Build history of the part. All positions in model axes, mm. A direction names the side the tool comes from. Coordinates: 2 decimals unless noted, no trailing zeros. Loops run counter-clockwise (first coordinate to the right, second up) from the corner with the lowest first, then second, coordinate; pieces in that order, holes last. Notation, with made-up numbers: M 10,10.5 L 23,10.5 A21 ccw 23,18.5 Z; hole C -27.75,69 d9. An arc over 180 degrees is marked long. Write each question's results on one line, items separated by ' | '. Start each with the question number.
from build123d import *

# Parameters (mm, degrees)
SKETCH1_W           = 120
SKETCH1_H           = 15
BOSS_EXTRUDE1_DEPTH = 5
SKETCH2_W           = 7
SKETCH2_H           = 4
CUT_EXTRUDE1_DEPTH  = 10
CUT_EXTRUDE2_DEPTH  = 7


with BuildPart() as part:
    # Sketch1 → Boss-Extrude1 (new body)
    with BuildSketch(Plane(origin=(0, 0, 0), x_dir=(1, 0, 0), z_dir=(0, 1, 0))):
        with Locations((60, 7.5)):
            Rectangle(SKETCH1_W, SKETCH1_H)
    extrude(amount=BOSS_EXTRUDE1_DEPTH)

    # Sketch2 → Cut-Extrude1 (cut)
    with BuildSketch(Plane(origin=(0, 5, 0), x_dir=(1, 0, 0), z_dir=(0, 1, 0))):
        with Locations((60, 7.5)):
            Rectangle(SKETCH2_W, SKETCH2_H)
    extrude(amount=-CUT_EXTRUDE1_DEPTH, mode=Mode.SUBTRACT)

    # Sketch3 → Cut-Extrude2 (cut)
    with BuildSketch(Plane(origin=(56.5, 0, 0), x_dir=(0, 0, -1), z_dir=(1, 0, 0))):
        Polygon((5.5, 5), (3.997858335, 5), (5.5, 2.5), align=None)
        Polygon((9.5, 5), (11, 5), (9.5, 2.5), align=None)
        Polygon((1.5, 5), (0, 2.5), (0, 5), align=None)
        Polygon((13.5, 5), (15, 2.5), (15, 5), align=None)
    extrude(amount=CUT_EXTRUDE2_DEPTH, mode=Mode.SUBTRACT)


solid = part.part
1. Band-saw the part on B-B, the plane y = 1.2. List the corners of the cut face in (x, z).
2. Which spindle directions (+Z, -Z, +X, -X, +Y, -Y) get a long thin tool onto all of the face, cutting with end or side? Do faces 1 (the flat face through (56.5, 3, -7)), 2 (the flat face through (60, 1, -5.5)), 3 (the flat face through (59.95, 3.77, -14.24)), 4 (the flat face through (120, 2, -7)), 5 (the flat face through (59.95, 3.77, -0.76)). Say none if no direction does.
3. Band-saw the part on A-A, the plane z = -8.5. List the corners of the cut face in (x, y).
4. Mould opens along X. For faces 6 (the flat face through (59, 2, -15)), 7 (the flat face through (59.95, 3.77, -10.26)), 8 (the flat face through (0, 2, -7)) say: +X half, -X half, draft (parallel to the pull), parting line (faces both ways), or undercut.
5. Wall check: line 1 along Z through (x, y) = (61, 1.05); line 2 along X through (y, z) = (3.25, -9.25); line 3 along Z through (x, y) = (59, 4.15). Give the ranges that are in metal, low to high.
Checked values:
1) outline: M 0,-15 L 120,-15 L 120,0 L 0,0 Z; hole M 56.5,-9.5 L 63.5,-9.5 L 63.5,-5.5 L 56.5,-5.5 Z
2) face 1: +Y | face 2: +Y, -Y | face 3: -Z, +Y | face 4: +Z, -Z, +X, +Y, -Y | face 5: +Z, +Y
3) outline: M 0,0 L 56.5,0 L 56.5,5 L 0,5 Z; M 63.5,0 L 120,0 L 120,5 L 63.5,5 Z
4) face 6: draft | face 7: undercut | face 8: -X half
5) line 1: -15 to -9.5, -5.5 to 0 | line 2: 0 to 56.5, 63.5 to 120 | line 3: -14.01 to -10.49, -4.51 to -0.99
